from build123d import *

# Parameters (mm, degrees)
F1_DEPTH = 12.7
F2_D     = 16.66748
F2_DEPTH = 12.7
F2_TIP   = 5.0074161752
F3_D     = 7.9375
F3_DEPTH = 17.4625
F3_TIP   = 2.3846655818


with BuildPart() as f1:
    # F0 (on Front) → F1 (new body)
    with BuildSketch(Plane.XZ):
        Polygon((177.8, 0), (482.6, 0), (482.6, 69.85), (469.8492, 69.85), (469.8492, 108.0516), (482.6, 108.0516), (482.6, 196.7484), (469.8492, 196.7484), (469.8492, 234.95), (482.6, 234.95), (482.6, 304.8), (177.8, 304.8), (177.8, 234.95), (190.5508, 234.95), (190.5508, 196.7484), (177.8, 196.7484), (177.8, 108.0516), (190.5508, 108.0516), (190.5508, 69.85), (177.8, 69.85), align=None)
    extrude(amount=F1_DEPTH)

    # F2
    with Locations(Plane(origin=(0, 0, 0), x_dir=(1, 0, 0), z_dir=(0, 1, 0))):
        with Locations((245.237, -274.32), (415.163, -274.32), (415.163, -90.17), (245.237, -90.17)):
            Hole(F2_D / 2, depth=F2_DEPTH)
            with Locations((0, 0, -(F2_DEPTH + F2_TIP / 2))):  # 118° drill point
                Cone(0, F2_D / 2, F2_TIP, mode=Mode.SUBTRACT)

    # F3
    with Locations(Plane(origin=(0, 0, 0), x_dir=(1, 0, 0), z_dir=(0, 1, 0))):
        with Locations((219.075, -279.4), (257.175, -207.9625), (219.075, -152.4), (403.225, -207.9625), (441.325, -279.4), (441.325, -152.4), (441.325, -25.4), (219.075, -25.4)):
            Hole(F3_D / 2, depth=F3_DEPTH)
            with Locations((0, 0, -(F3_DEPTH + F3_TIP / 2))):  # 118° drill point
                Cone(0, F3_D / 2, F3_TIP, mode=Mode.SUBTRACT)


solid = f1.part
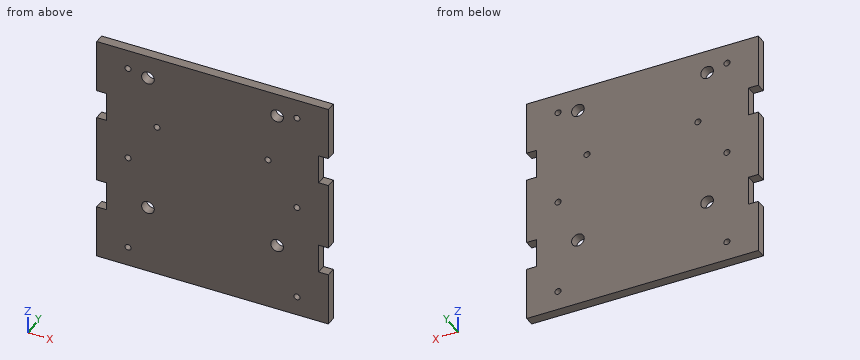
The model under review builds one solid part; all positions refer to its coordinate system, in mm. Round coordinates to 2 decimals unless told otherwise and drop trailing zeros. Write each loop counter-clockwise with the first axis right and the second up, starting at its lowest first coordinate (ties: lowest second). Pieces come first, ordered by that corner, then holes. Notation, with made-up numbers: (-13.75, -17.5) -> (4.25, -17.5) arc R16 ccw to (4.25, 5.5) -> close; hole circle Ø7 at (-21.75, 61). An arc over 180 degrees is marked (long way). Answer as a JSON object with one key per item and string values.
1. We need section A-A on z = 152.4. State the section outline as (x, y) points, and give its area (3 significant figures).
Results found:
{"outline": "(177.8, -12.7) -> (215.11, -12.7) -> (215.11, 0) -> (177.8, 0) -> close; (223.04, -12.7) -> (437.36, -12.7) -> (437.36, 0) -> (223.04, 0) -> close; (445.29, -12.7) -> (482.6, -12.7) -> (482.6, 0) -> (445.29, 0) -> close", "area": "3,670 mm^2"}
2. We need section D-D on z = 221.5. State the section outline as (x, y) points, and give its area (3 significant figures).
Results found:
{"outline": "(190.55, -12.7) -> (469.85, -12.7) -> (469.85, 0) -> (190.55, 0) -> close", "area": "3,550 mm^2"}
3. Clearance check with flat-ended pins moving along their axes: pin 1 (4 mm diameter, centred on y = -3.5, z = 217.5, fed in from -X); pin 2 (12.5 mm diameter, centred on x = 441.325, z = 152.4, fed in from -Y). State where each tip first meets the part, or that it passes through.
Results found:
{"pin 1": "stops at x = 190.55", "pin 2": "stops at y = -12.7"}
4. We need section B-B on x = 416. State the section outline as (y, z) points.
Results found:
{"outline": "(-12.7, 0) -> (0, 0) -> (0, 81.88) -> (-12.7, 81.88) -> close; (-12.7, 98.46) -> (0, 98.46) -> (0, 266.03) -> (-12.7, 266.03) -> close; (-12.7, 282.61) -> (0, 282.61) -> (0, 304.8) -> (-12.7, 304.8) -> close"}
5. To check wall thickness, follow line 1 along X through (y, z) = (-6.25, 90.17); line 2 along X through (y, z) = (-4.75, 25.4); line 3 along Z through (x, y) = (256.5, -10). State the ranges of each line that lie inside material, in increasing order.
Results found:
{"line 1": "x = 190.55 to 236.9, 253.57 to 406.83, 423.5 to 469.85", "line 2": "x = 177.8 to 215.11, 223.04 to 437.36, 445.29 to 482.6", "line 3": "z = 0 to 204.05, 211.87 to 304.8"}
6. We need section C-C on y = -5.5. State how many separate pieces and enclosed holes the cut face has, and give its area (3 significant figures).
Results found:
{"separate pieces": "1", "enclosed holes": "12", "area": "89,700 mm^2"}
